Could you check a few things on this drawing? It's one solid part, dimensions in mm from its lowest x, y, z. Coordinates: 2 decimals unless noted, no trailing zeros. Order: outer loops, then holes, each group sorted by start corner. A loop starts at its lowest first (then second) coordinate and runs counter-clockwise, first axis right, second up. Notation, with made-up numbers: (23.25, -31.5) -> (57.25, -31.5) arc R26 cw to (57.25, -16.5) -> close; hole circle Ø4 at (-29, -38). An arc over 180 degrees is marked (long way). Answer as CSV lines item,"result".
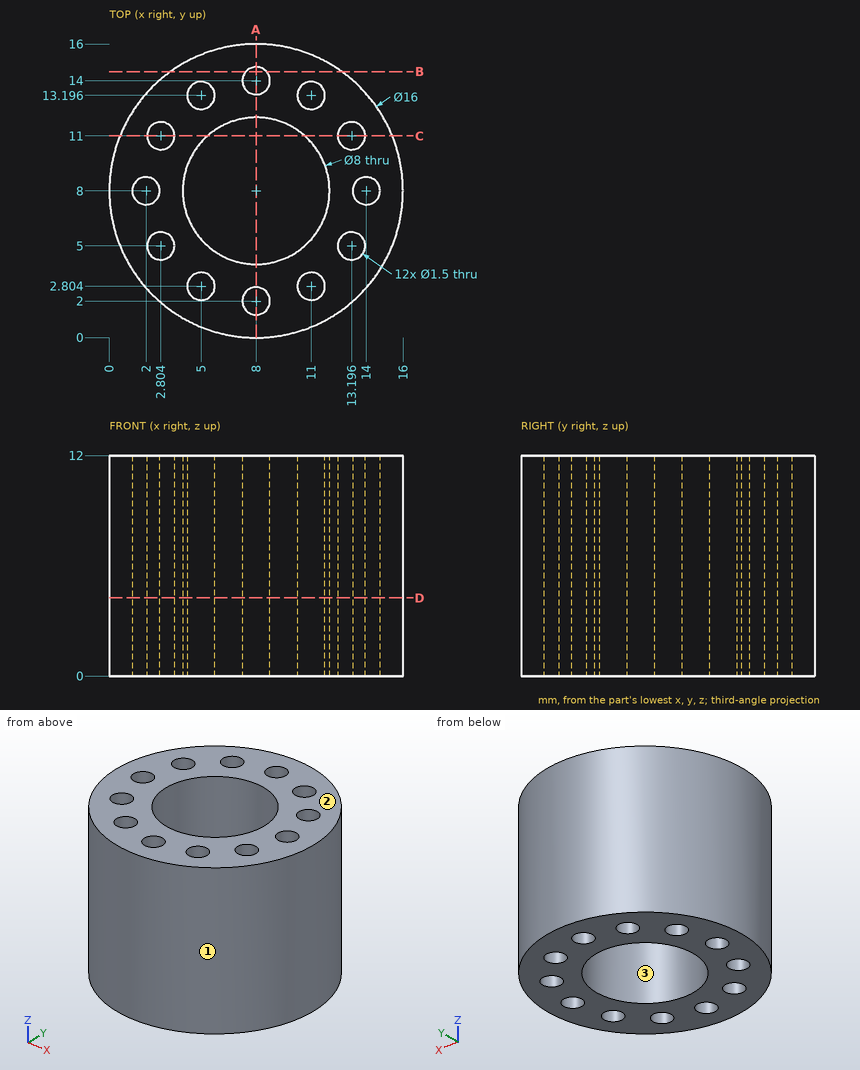
Q1. Imagine slicing it at B-B (y = 14.5). List the corners of the cut face in (x, z) for me.
Solution:
outline,"(3.34, 0) -> (7.44, 0) -> (7.44, 12) -> (3.34, 12) -> close; (8.56, 0) -> (12.66, 0) -> (12.66, 12) -> (8.56, 12) -> close"
Q2. Imagine slicing it at A-A (x = 8). List the corners of the cut face in (y, z) for me, and give its area (3 significant figures).
Solution:
outline,"(0, 0) -> (1.25, 0) -> (1.25, 12) -> (0, 12) -> close; (2.75, 0) -> (4, 0) -> (4, 12) -> (2.75, 12) -> close; (12, 0) -> (13.25, 0) -> (13.25, 12) -> (12, 12) -> close; (14.75, 0) -> (16, 0) -> (16, 12) -> (14.75, 12) -> close"
area,"60.0 mm2"
Q3. If I drill on line 1 (Y direction, x = 7.75, z = 4.25); line 2 (Y direction, x = 2.5, z = 5.75) (1 decimal); line 3 (X direction, y = 10.5, z = 7) (1 decimal), over which ranges is the centre line in solid material (lowest first)?
Solution:
line 1,"0 to 1.29, 2.71 to 4.01, 11.99 to 13.29, 14.71 to 16"
line 2,"2.2 to 4.3, 5.7 to 7.4, 8.6 to 10.3, 11.7 to 13.8"
line 3,"0.4 to 2.2, 3.4 to 4.9, 11.1 to 12.6, 13.8 to 15.6"
Q4. Imagine slicing it at D-D (z = 4.25). Give the number of separate pieces and of enclosed holes in the cut face, and give its area (3 significant figures).
Solution:
separate pieces,"1"
enclosed holes,"13"
area,"130 mm2"
Q5. We'd pull the mould along Y, two halves only. Please class the marked faces 1, 2 and 3: pulls with the +Y half, pulls with the -Y half, needs draft (parallel to the pull), parting line crosses it, or undercut.
Solution:
face 1,"parting line crosses it"
face 2,"needs draft"
face 3,"undercut"
Q6. Imagine slicing it at C-C (y = 11). List the corners of the cut face in (x, z) for me.
Solution:
outline,"(0.58, 0) -> (2.05, 0) -> (2.05, 12) -> (0.58, 12) -> close; (3.55, 0) -> (5.35, 0) -> (5.35, 12) -> (3.55, 12) -> close; (10.65, 0) -> (12.45, 0) -> (12.45, 12) -> (10.65, 12) -> close; (13.95, 0) -> (15.42, 0) -> (15.42, 12) -> (13.95, 12) -> close"
Q7. For P1, Ø1.5, axis at y = 9, z = 5.5, coming from the +X side; P2, Ø5, axis at y = 14, z = 4.5, coming from the +X side; P3, Ø1.5, axis at x = 10.5, z = 10.5, coming from the +Y side, each with a flat end and sliding along its axis, tell me the tip position at first contact or that it passes through.
Solution:
P1,"x = 16"
P2,"x = 15.19"
P3,"y = 15.81"
